```python
from build123d import *

# Parameters (mm, degrees)
SKETCH1_W           = 2050
SKETCH1_H           = 300
BOSS_EXTRUDE1_DEPTH = 25
CUT_EXTRUDE1_REACH  = 2073.986
SKETCH2_W           = 90
SKETCH2_H           = 90


with BuildPart() as part:
    # Sketch1 → Boss-Extrude1 (new body)
    with BuildSketch(Plane(origin=(0, 0, 0), x_dir=(1, 0, 0), z_dir=(0, 1, 0))):
        with Locations((1025, 150)):
            Rectangle(SKETCH1_W, SKETCH1_H)
    extrude(amount=BOSS_EXTRUDE1_DEPTH)

    # Sketch2 → Cut-Extrude1 (cut, up to next)
    with BuildSketch(Plane(origin=(0, 25, 0), x_dir=(1, 0, 0), z_dir=(0, 1, 0)), mode=Mode.PRIVATE) as cut_extrude1_sk1:
        with Locations((470, 45)):
            Rectangle(SKETCH2_W, SKETCH2_H)
    cut_extrude1_tool1 = extrude(cut_extrude1_sk1.sketch, amount=-CUT_EXTRUDE1_REACH, mode=Mode.PRIVATE) & part.part
    # Sketch2 → Cut-Extrude1 (cut, up to next)
    with BuildSketch(Plane(origin=(0, 25, 0), x_dir=(1, 0, 0), z_dir=(0, 1, 0)), mode=Mode.PRIVATE) as cut_extrude1_sk2:
        with Locations((1580, 45)):
            Rectangle(SKETCH2_W, SKETCH2_H)
    cut_extrude1_tool2 = extrude(cut_extrude1_sk2.sketch, amount=-CUT_EXTRUDE1_REACH, mode=Mode.PRIVATE) & part.part
    add(cut_extrude1_tool1.solids().sort_by_distance((470, 25, -45))[0], mode=Mode.SUBTRACT)
    add(cut_extrude1_tool2.solids().sort_by_distance((1580, 25, -45))[0], mode=Mode.SUBTRACT)


solid = part.part
```
Verification items for the finished model (mm, model axes). Coordinates: 2 decimals unless noted, no trailing zeros. Order: outer loops, then holes, each group sorted by start corner. A loop starts at its lowest first (then second) coordinate and runs counter-clockwise, first axis right, second up. Notation, with made-up numbers: (80.5, 23.25) - (94.5, 23.25) arc R22 ccw to (94.5, 33.25) - close; hole circle Ø6 at (-40, 19.25). An arc over 180 degrees is marked (long way). Return JSON: item names as keys, results as strings.
(1) Go/stop test with flat-tipped pins: pin 1 (8 mm diameter, centred on x = 1201.5, y = 5, fed in from +Z); pin 2 (12.5 mm diameter, centred on x = 1578, y = 15, fed in from +Z). Record where each tip stops, or that it passes through.
Filled sheet:
{"pin 1": "stops at z = 0", "pin 2": "stops at z = -90"}
(2) Thickness scan on line 1 along X through (y, z) = (12.75, -51); line 2 along Z through (x, y) = (1612, 4). Record the ranges inside material, lowest first.
Filled sheet:
{"line 1": "x = 0 to 425, 515 to 1535, 1625 to 2050", "line 2": "z = -300 to -90"}
(3) Section check A-A, the plane y = 12.75. Record the cut outline in (x, z).
Filled sheet:
{"outline": "(0, -300) - (2050, -300) - (2050, 0) - (1625, 0) - (1625, -90) - (1535, -90) - (1535, 0) - (515, 0) - (515, -90) - (425, -90) - (425, 0) - (0, 0) - close"}
